Check sheet for the modelled part. Datum: model origin and axes. Units: mm. Face numbers are marked on the shaded views. A direction names the side the tool comes from. Coordinates: 2 decimals unless noted, no trailing zeros. Loops run counter-clockwise (first coordinate to the right, second up) from the corner with the lowest first, then second, coordinate; pieces in that order, holes last. Notation, with made-up numbers: (23.25, 85) -> (64.25, 85) arc R21 cw to (64.25, 104) -> close; hole circle Ø2 at (-39, 68.25). An arc over 180 degrees is marked (long way). Use CSV: the item, a comma, the result in double quotes.
Autodesk Inventor part; units mm, degrees
ref_plane "YZ Plane" through (0, 0, 0) normal (1, 0, 0) x (0, 1, 0)
ref_plane "XZ Plane" through (0, 0, 0) normal (0, 1, 0) x (-1, 0, 0)
ref_plane "XY Plane" through (0, 0, 0) normal (0, 0, 1) x (1, 0, 0)
sketch "Sketch1" plane through (0, 0, 0) normal (0, 1, 0) x (-1, 0, 0)
  line L0 (8.2561, 0) -> (4.1281, -7.15)
  line L1 (4.1281, -7.15) -> (-4.1281, -7.15)
  line L2 (-4.1281, -7.15) -> (-8.2561, 0)
  line L3 (-8.2561, 0) -> (-4.1281, 7.15)
  line L4 (-4.1281, 7.15) -> (4.1281, 7.15)
  line L5 (4.1281, 7.15) -> (8.2561, 0)
  point P0 (0, 0)
  point P1 (0, 0)
  dimension "d0" = 14.3
extrude "Extrusion1" add sketch "Sketch1" along normal blind 6.35
sketch "Sketch2" plane through (0, 6.35, 0) normal (0, 1, 0) x (1, 0, 0)
  circle A0 centre (0, 0) radius 7.15
  dimension "d3" = 14.3
extrude "Extrusion2" cut sketch "Sketch2" against normal through all draft 45 keep common part
sketch "Sketch3" plane through (0, 0, 0) normal (0, -1, 0) x (1, 0, 0)
  circle A0 centre (0, 0) radius 4.765
  dimension "d6" = 9.53
extrude "Extrusion3" add sketch "Sketch3" along normal blind 20.32
chamfer "Chamfer1" distance 1 angle 45 1 edges at (-4.765, -20.32, 0)
fillet "Fillet1" radius 1 1 edges at (-4.765, 0, 0)
thread "Thread1"
properties part number "Bolt" material "Stainless Steel"
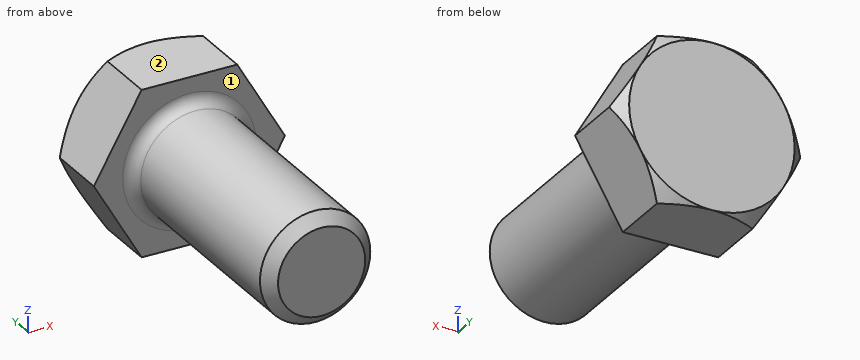
1) Cross-section at B-B on y = -0.5. Record the boundary of the cut face in (x, z), and give its area (3 significant figures).
Answer below:
outline,"circle Ø9.8 at (0, 0)"
area,"75.4 mm²"
2) Access from +Z, -Z, +X, -X, +Y, -Y to the whole of each face (thin tool, end or side, straight path). Record for the marked faces 1 and 2.
Answer below:
face 1,"-Y"
face 2,"+Z, +X, -X, +Y, -Y"
3) Thickness scan on line 1 along Y through (x, z) = (-0.75, -6.25); line 2 along X through (y, z) = (-19, 3.75); line 3 along Z through (x, y) = (0.25, -16.25). Record the ranges inside material, lowest first. Write a range as from..to.
Answer below:
line 1,"y = 0..6.35"
line 2,"x = -2.94..2.94"
line 3,"z = -4.76..4.76"
4) Go/stop test with flat-tipped pins: pin 1 Ø5 at (x, y) = (0.5, -7) entering from -Z (3 decimals); pin 2 Ø3 at (y, z) = (2, 3.5) entering from +X; pin 3 Ø1 at (y, z) = (-8.5, -1.5) entering from +X. Record where each tip stops, or that it passes through.
Answer below:
pin 1,"stops at z = -4.765"
pin 2,"stops at x = 7.1"
pin 3,"stops at x = 4.66"
5) Cross-section at A-A on y = -16.5. Record the boundary of the cut face in (x, z) (3 decimals).
Answer below:
outline,"circle Ø9.53 at (0, 0)"
